```python
from build123d import *

# Parameters (mm, degrees)
BOSS_EXTRUDE1_DEPTH = 0.79375
FILLET2_R           = 6.35
FILLET3_R           = 3.175


with BuildPart() as part:
    # Sketch1 → Boss-Extrude1 (new body, symmetric)
    with BuildSketch(Plane(origin=(0, 0, 0), x_dir=(1, 0, 0), z_dir=(0, 1, 0))):
        Polygon((-71.12, 101.9175), (-25.4, 101.9175), (-25.4, 100.33), (25.4, 100.33), (25.4, 101.9175), (71.12, 101.9175), (71.12, 25.4), (59.182, 25.4), (59.182, -25.4), (71.12, -25.4), (71.12, -101.9175), (25.4, -101.9175), (25.4, -100.33), (-25.4, -100.33), (-25.4, -101.9175), (-71.12, -101.9175), (-71.12, -25.4), (-59.182, -25.4), (-59.182, 25.4), (-71.12, 25.4), align=None)
    extrude(amount=BOSS_EXTRUDE1_DEPTH, both=True)

    # Fillet2
    fillet2_edges = [part.edges().sort_by_distance(p)[0] for p in [
        (59.182, 0, -25.4),
        (59.182, 0, 25.4),
        (-59.182, 0, 25.4),
        (-59.182, 0, -25.4),
    ]]
    fillet(fillet2_edges, radius=FILLET2_R)

    # Fillet3
    fillet3_edges = [part.edges().sort_by_distance(p)[0] for p in [
        (71.12, 0, -25.4),
        (71.12, 0, 25.4),
        (-71.12, 0, 25.4),
        (-71.12, 0, -25.4),
    ]]
    fillet(fillet3_edges, radius=FILLET3_R)


solid = part.part
```
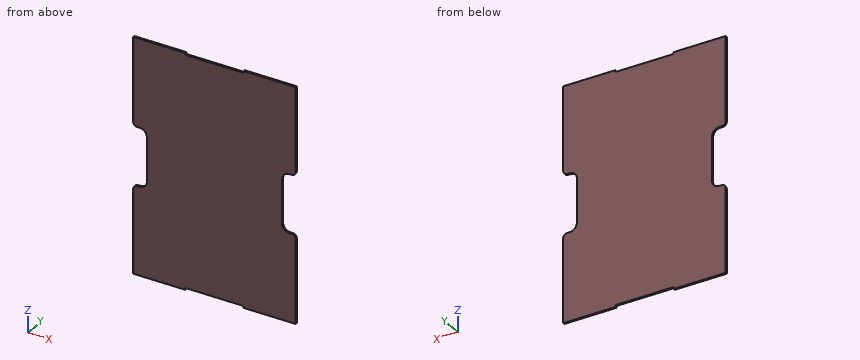
Input: part model. Units: mm. Frame: model coordinates. Coordinates: 2 decimals unless noted, no trailing zeros. Write each loop counter-clockwise with the first axis right and the second up, starting at its lowest first coordinate (ties: lowest second). Pieces come first, ordered by that corner, then holes.
1) Pin query (flat end, axial travel): pin 1 Ø0.5 at (x, y) = (-8, 0) entering from +Z; pin 2 Ø0.8 at (x, y) = (-2, 0) entering from -Z. Return the tip coordinate at first contact, or that it passes through.
2) Section C-C on z = 6. Output: boundary loops of the cut face in (x, y), and give its area (3 significant figures).
3) Section B-B on x = 17.5. Output: boundary loops of the cut face in (y, z), and give its area (3 significant figures).
4) Material intervals for line 1 along Z through (x, y) = (11.5, 0.1); line 2 along X through (y, z) = (0.6, -16); line 3 along Z through (x, y) = (-63, -0.55), sorted ascending.
Check result:
1. pin 1: stops at z = 100.33
1. pin 2: stops at z = -100.33
2. outline: (-59.18, -0.79) - (59.18, -0.79) - (59.18, 0.79) - (-59.18, 0.79) - close
2. area: 188 mm2
3. outline: (-0.79, -100.33) - (0.79, -100.33) - (0.79, 100.33) - (-0.79, 100.33) - close
3. area: 319 mm2
4. line 1: z = -100.33 to 100.33
4. line 2: x = -59.18 to 59.18
4. line 3: z = -101.92 to -24.87, 24.87 to 101.92
